from build123d import *

# Parameters (mm, degrees)
SKETCH_1_W          = 120
SKETCH_1_H          = 100
EXTRUDE_1_DEPTH     = 5
SKETCH_2_W          = 3
SKETCH_2_H          = 100
CUT_EXTRUDE_1_DEPTH = 2
SKETCH_3_R          = 1.75
SKETCH_3_W          = 80
SKETCH_3_H          = 44
SKETCH_3_H_2        = 9
SKETCH_3_W_2        = 59
SKETCH_3_H_3        = 19
CUT_EXTRUDE_2_DEPTH = 157.284996081


with BuildPart() as part:
    # 草图1 → 凸台-拉伸1 (new body)
    with BuildSketch(Plane.XY):
        with Locations((60, 50)):
            Rectangle(SKETCH_1_W, SKETCH_1_H)
    extrude(amount=EXTRUDE_1_DEPTH)

    # 草图2 → 切除-拉伸1 (cut)
    with BuildSketch(Plane.XY.offset(5)):
        with Locations((10.45, 50)):
            Rectangle(SKETCH_2_W, SKETCH_2_H)
        with Locations((109.55, 50)):
            Rectangle(SKETCH_2_W, SKETCH_2_H)
    extrude(amount=-CUT_EXTRUDE_1_DEPTH, mode=Mode.SUBTRACT)

    # 草图3 → 切除-拉伸2 (cut, through all)
    with BuildSketch(Plane.XY.offset(5)):
        with Locations((20.5, 80)):
            Circle(SKETCH_3_R)
        with Locations((20.5, 61)):
            Circle(SKETCH_3_R)
        with Locations((99.5, 80)):
            Circle(SKETCH_3_R)
        with Locations((99.5, 61)):
            Circle(SKETCH_3_R)
        with Locations((60, 29)):
            Rectangle(SKETCH_3_W, SKETCH_3_H)
        with Locations((60, 91.5)):
            Rectangle(SKETCH_3_W, SKETCH_3_H_2)
        with Locations((60, 70.5)):
            Rectangle(SKETCH_3_W_2, SKETCH_3_H_3)
    extrude(amount=-CUT_EXTRUDE_2_DEPTH, mode=Mode.SUBTRACT)


solid = part.part
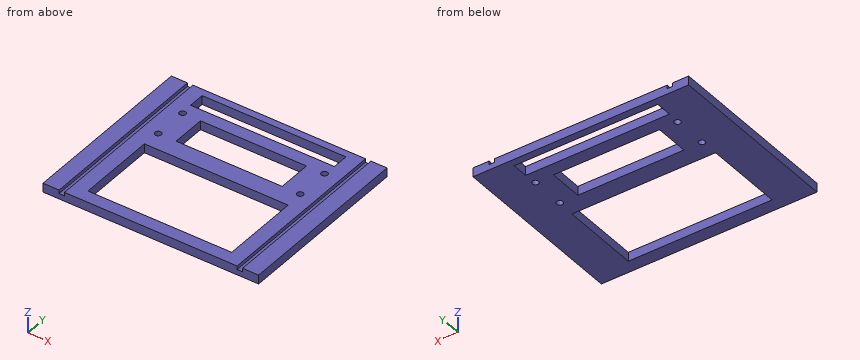
Build history of the part. All positions in model axes, mm. Round coordinates to 2 decimals unless told otherwise and drop trailing zeros. Loops run counter-clockwise (first coordinate to the right, second up) from the corner with the lowest first, then second, coordinate; pieces in that order, holes last. Notation, with made-up numbers: (26.5, 8) -> (70.5, 8) arc R20 ccw to (70.5, 19) -> close; hole circle Ø1 at (30, -17). An arc over 180 degrees is marked (long way). Answer in a Markdown table with one row per item.
Item 1: Saw through at C-C (z = 2). Write the cut outline in (x, y), and give its area (3 significant figures).
Answers below:
| item | result |
|---|---|
| outline | (0, 0) -> (120, 0) -> (120, 100) -> (0, 100) -> close; hole circle Ø3.5 at (20.5, 61); hole circle Ø3.5 at (20.5, 80); hole (20, 7) -> (100, 7) -> (100, 51) -> (20, 51) -> close; hole (20, 87) -> (100, 87) -> (100, 96) -> (20, 96) -> close; hole (30.5, 61) -> (89.5, 61) -> (89.5, 80) -> (30.5, 80) -> close; hole circle Ø3.5 at (99.5, 61); hole circle Ø3.5 at (99.5, 80) |
| area | 6,600 mm² |
Item 2: Drill centre lines: L1, parallel to Y at x = 99.5, z = 1.25; L2, parallel to X at y = 30, z = 3.4; L3, parallel to Y at x = 52, z = 2.6. Where is each one in solid material? Low to high. Write a range as [from, to].
Answers below:
| item | result |
|---|---|
| L1 | y = [0, 7], [51, 59.25], [62.75, 78.25], [81.75, 87], [96, 100] |
| L2 | x = [0, 8.95], [11.95, 20], [100, 108.05], [111.05, 120] |
| L3 | y = [0, 7], [51, 61], [80, 87], [96, 100] |
Item 3: Saw through at A-A (y = 35.5). Write the cut outline in (x, z), and give its area (3 significant figures).
Answers below:
| item | result |
|---|---|
| outline | (0, 0) -> (20, 0) -> (20, 5) -> (11.95, 5) -> (11.95, 3) -> (8.95, 3) -> (8.95, 5) -> (0, 5) -> close; (100, 0) -> (120, 0) -> (120, 5) -> (111.05, 5) -> (111.05, 3) -> (108.05, 3) -> (108.05, 5) -> (100, 5) -> close |
| area | 188 mm² |
Item 4: Saw through at D-D (y = 76.5). Write the cut outline in (x, z), and give its area (3 significant figures).
Answers below:
| item | result |
|---|---|
| outline | (0, 0) -> (30.5, 0) -> (30.5, 5) -> (11.95, 5) -> (11.95, 3) -> (8.95, 3) -> (8.95, 5) -> (0, 5) -> close; (89.5, 0) -> (120, 0) -> (120, 5) -> (111.05, 5) -> (111.05, 3) -> (108.05, 3) -> (108.05, 5) -> (89.5, 5) -> close |
| area | 293 mm² |
Item 5: Saw through at B-B (x = 42.5). Write the cut outline in (y, z).
Answers below:
| item | result |
|---|---|
| outline | (0, 0) -> (7, 0) -> (7, 5) -> (0, 5) -> close; (51, 0) -> (61, 0) -> (61, 5) -> (51, 5) -> close; (80, 0) -> (87, 0) -> (87, 5) -> (80, 5) -> close; (96, 0) -> (100, 0) -> (100, 5) -> (96, 5) -> close |
